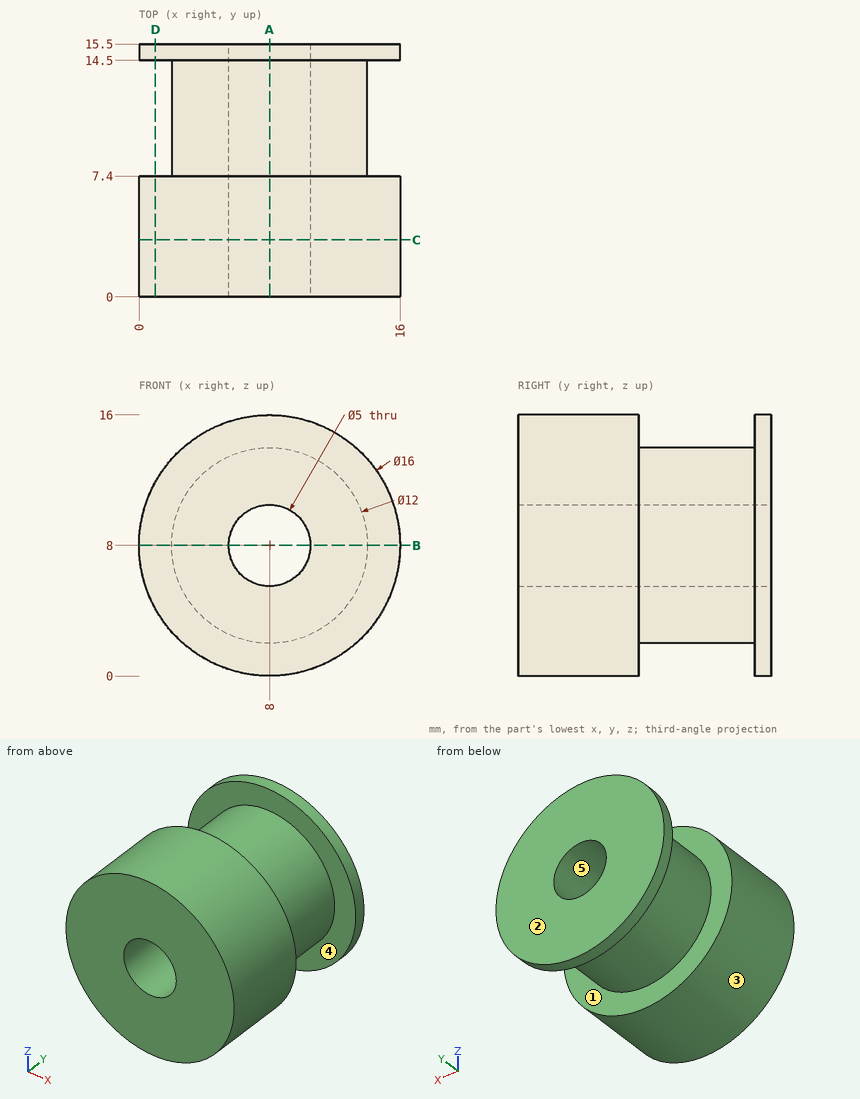
Check sheet for the drawn part. Datum: minimum x, y, z corner. Units: mm. A direction names the side the tool comes from. Coordinates: 2 decimals unless noted, no trailing zeros. Loops run counter-clockwise (first coordinate to the right, second up) from the corner with the lowest first, then second, coordinate; pieces in that order, holes last. Notation, with made-up numbers: (42.25, 83) -> (79.25, 83) arc R35 ccw to (79.25, 117) -> close; hole circle Ø6 at (34, -24.5). An arc over 180 degrees is marked (long way). Answer in a Markdown table with one row per item.
1. Access from +Z, -Z, +X, -X, +Y, -Y to the whole of each face (thin tool, end or side, straight path). Record for the marked faces 1 and 2.
Check values:
| item | result |
|---|---|
| face 1 | none |
| face 2 | +Z, -Z, +X, -X, +Y |
2. Sectioned sample at A-A, the plane x = 8. Record the boundary of the cut face in (y, z), then the cut area to 3 significant figures.
Check values:
| item | result |
|---|---|
| outline | (0, 0) -> (7.4, 0) -> (7.4, 2) -> (14.5, 2) -> (14.5, 0) -> (15.5, 0) -> (15.5, 5.5) -> (0, 5.5) -> close; (0, 10.5) -> (15.5, 10.5) -> (15.5, 16) -> (14.5, 16) -> (14.5, 14) -> (7.4, 14) -> (7.4, 16) -> (0, 16) -> close |
| area | 142 mm2 |
3. Sectioned sample at D-D, the plane x = 1. Record the boundary of the cut face in (y, z), then the cut area to 3 significant figures.
Check values:
| item | result |
|---|---|
| outline | (0, 4.13) -> (7.4, 4.13) -> (7.4, 11.87) -> (0, 11.87) -> close; (14.5, 4.13) -> (15.5, 4.13) -> (15.5, 11.87) -> (14.5, 11.87) -> close |
| area | 65.1 mm2 |
4. Material ranges on line 1 along Z through (x, y) = (8, 5.5); line 2 along Y through (x, z) = (4.5, 1); line 3 along X through (y, z) = (11.75, 8), recorded low to high. Write a range as [from, to].
Check values:
| item | result |
|---|---|
| line 1 | z = [0, 5.5], [10.5, 16] |
| line 2 | y = [0, 7.4], [14.5, 15.5] |
| line 3 | x = [2, 5.5], [10.5, 14] |
5. Sectioned sample at C-C, the plane y = 3.5. Record the boundary of the cut face in (x, z), then the cut area to 3 significant figures.
Check values:
| item | result |
|---|---|
| outline | circle Ø16 at (8, 8); hole circle Ø5 at (8, 8) |
| area | 181 mm2 |
6. Sectioned sample at B-B, the plane z = 8. Record the boundary of the cut face in (x, y), then the cut area to 3 significant figures.
Check values:
| item | result |
|---|---|
| outline | (0, 0) -> (5.5, 0) -> (5.5, 15.5) -> (0, 15.5) -> (0, 14.5) -> (2, 14.5) -> (2, 7.4) -> (0, 7.4) -> close; (10.5, 0) -> (16, 0) -> (16, 7.4) -> (14, 7.4) -> (14, 14.5) -> (16, 14.5) -> (16, 15.5) -> (10.5, 15.5) -> close |
| area | 142 mm2 |
7. Release check for a two-part mould opening along X. For the marked faces 3, 4 and 5 record: released by +X, released by -X, zero draft, split by the parting line, or undercut.
Check values:
| item | result |
|---|---|
| face 3 | split by the parting line |
| face 4 | zero draft |
| face 5 | undercut |
8. Go/stop test with flat-tipped pins: pin 1 (6 mm diameter, centred on y = 10.5, z = 11, fed in from +X); pin 2 (8 mm diameter, centred on y = 7, z = 13.5, fed in from +X); pin 3 (3 mm diameter, centred on y = 10, z = 11.5, fed in from +X). Record where each tip stops, or that it passes through.
Check values:
| item | result |
|---|---|
| pin 1 | stops at x = 14 |
| pin 2 | stops at x = 15.86 |
| pin 3 | stops at x = 13.66 |
